Can you work these out from the model? Positions are in its coordinate system, mm. Face numbers are marked on the shaded views. Coordinates: 2 decimals unless noted, no trailing zeros. Order: outer loops, then holes, each group sorted by start corner. A loop starts at its lowest first (then second) coordinate and runs counter-clockwise, first axis right, second up. Notation, with made-up numbers: (0, 12) -> (29, 12) arc R17 ccw to (29, 16) -> close; hole circle Ø2 at (45.5, 26). An arc over 180 degrees is marked (long way). Answer in a Markdown table with one row per item. Add a question column.
1. Will these pins go through, and if not, where does the flat tip stop? pin 1 (1 mm diameter, centred on y = 0, z = -10, fed in from -X); pin 2 (1.5 mm diameter, centred on x = 3.5, y = 1, fed in from -Z).
2. Imagine slicing it at B-B on z = 0.5. Write out the boundary of the cut face in (x, y).
3. Imagine slicing it at A-A on x = 0. Write out the boundary of the cut face in (y, z).
4. We'd pull the mould along X, two halves only. Please class the marked faces 1, 2 and 3: pulls with the +X half, pulls with the -X half, needs draft (parallel to the pull), parting line crosses it, or undercut.
5. Imagine slicing it at C-C on y = -0.9. Write out the boundary of the cut face in (x, z).
6. Imagine slicing it at D-D on x = -3. Write out the boundary of the cut face in (y, z).
7. If I drill on line 1 along Z through (x, y) = (0, -0.4); line 2 along X through (y, z) = (-0.55, 0); line 3 along Z through (x, y) = (2.5, 0.55), over which ranges is the centre line in solid material (lowest first)? Write a range as [from, to].
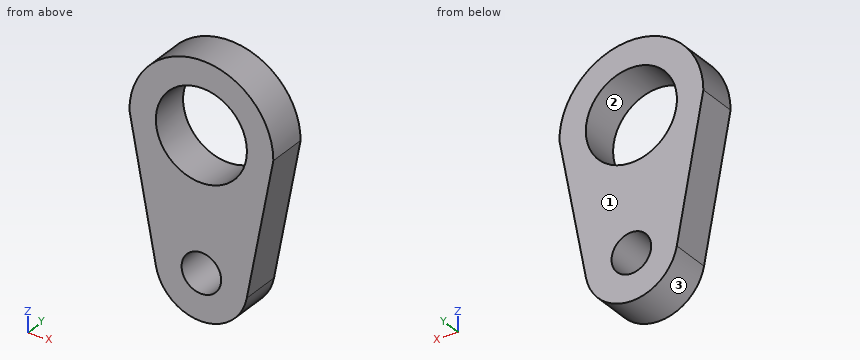
from build123d import *

# Parameters (mm, degrees)
SKETCH1_R           = 3.45
SKETCH1_R_2         = 1.5
BOSS_EXTRUDE1_DEPTH = 1.5


with BuildPart() as part:
    # Sketch1 → Boss-Extrude1 (new body, symmetric)
    with BuildSketch(Plane(origin=(0, 0, 0), x_dir=(1, 0, 0), z_dir=(0, 1, 0))):
        with BuildLine():
            Line((-5.45, 0), (-3.439230286, 10.649380506))
            ThreePointArc((-3.439230286, 10.649380506), (0, 13.5), (3.439230286, 10.649380506))
            Line((3.439230286, 10.649380506), (5.45, 0))
            ThreePointArc((5.45, 0), (0, -5.45), (-5.45, 0))
        make_face()
        Circle(SKETCH1_R, mode=Mode.SUBTRACT)
        with Locations((0, 10)):
            Circle(SKETCH1_R_2, mode=Mode.SUBTRACT)
    extrude(amount=BOSS_EXTRUDE1_DEPTH, both=True)


solid = part.part
Answers follow:
| question | item | result |
|---|---|---|
| 1 | pin 1 | stops at x = -3.66 |
| 1 | pin 2 | stops at z = -12.17 |
| 2 | outline | (-5.43, -1.5) -> (-3.41, -1.5) -> (-3.41, 1.5) -> (-5.43, 1.5) -> close; (3.41, -1.5) -> (5.43, -1.5) -> (5.43, 1.5) -> (3.41, 1.5) -> close |
| 3 | outline | (-1.5, -13.5) -> (1.5, -13.5) -> (1.5, -11.5) -> (-1.5, -11.5) -> close; (-1.5, -8.5) -> (1.5, -8.5) -> (1.5, -3.45) -> (-1.5, -3.45) -> close; (-1.5, 3.45) -> (1.5, 3.45) -> (1.5, 5.45) -> (-1.5, 5.45) -> close |
| 4 | face 1 | needs draft |
| 4 | face 2 | undercut |
| 4 | face 3 | parting line crosses it |
| 5 | outline | (-5.45, 0) -> (-3.44, -10.65) arc R3.5 ccw to (3.44, -10.65) -> (5.45, 0) arc R5.45 ccw to start; hole circle Ø6.9 at (0, 0); hole circle Ø3 at (0, -10) |
| 6 | outline | (-1.5, -11.8) -> (1.5, -11.8) -> (1.5, -1.7) -> (-1.5, -1.7) -> close; (-1.5, 1.7) -> (1.5, 1.7) -> (1.5, 4.55) -> (-1.5, 4.55) -> close |
| 7 | line 1 | z = [-13.5, -11.5], [-8.5, -3.45], [3.45, 5.45] |
| 7 | line 2 | x = [-5.45, -3.45], [3.45, 5.45] |
| 7 | line 3 | z = [-12.45, -2.38], [2.38, 4.84] |
